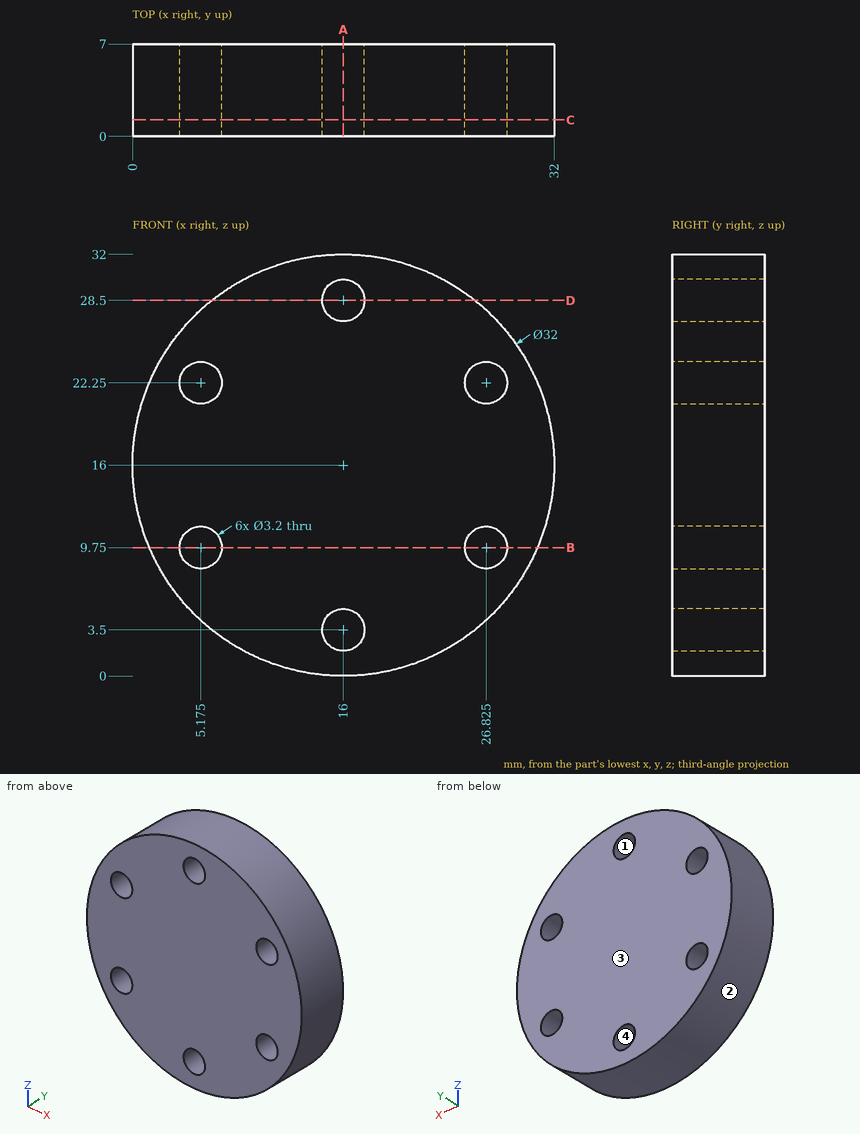
Source: three-view drawing plus pictorial views. Frame: mm from the lowest corner of the part. Give positions to 0.01 mm unless a question says otherwise; leave off trailing zeros. Write each loop counter-clockwise with the first axis right and the second up, starting at its lowest first coordinate (ties: lowest second). Pieces come first, ordered by that corner, then holes. Notation, with made-up numbers: (8, 38) -> (33, 38) arc R25 ccw to (33, 56) -> close; hole circle Ø5 at (-30, -8.75). An arc over 180 degrees is marked (long way). Answer in a Markdown table with one row per item.
(1) Ray query, line 1 along Z through (x, y) = (4.5, 5.25) (1 decimal); line 2 along Z through (x, y) = (26, 5); line 3 along X through (y, z) = (5.25, 4) (1 decimal). Return the intervals inside material, ascending. Write a range as [from, to].
Answers below:
| item | result |
|---|---|
| line 1 | [4.9, 8.3], [11.2, 20.8], [23.7, 27.1] |
| line 2 | [3.51, 8.38], [11.12, 20.88], [23.62, 28.49] |
| line 3 | [5.4, 14.5], [17.5, 26.6] |
(2) Section query D-D on z = 28.5. Return loops of the section in (x, y).
Answers below:
| item | result |
|---|---|
| outline | (6.01, 0) -> (14.4, 0) -> (14.4, 7) -> (6.01, 7) -> close; (17.6, 0) -> (25.99, 0) -> (25.99, 7) -> (17.6, 7) -> close |
(3) Draft query along Z for the marked faces 1, 2, 3 and 4. Return one class per face: +Z half, -Z half, draft (parallel to the pull), parting line (faces both ways), or undercut.
Answers below:
| item | result |
|---|---|
| face 1 | undercut |
| face 2 | parting line |
| face 3 | draft |
| face 4 | undercut |
(4) Section query A-A on x = 16. Return loops of the section in (y, z), then the cut area to 3 significant figures.
Answers below:
| item | result |
|---|---|
| outline | (0, 0) -> (7, 0) -> (7, 1.9) -> (0, 1.9) -> close; (0, 5.1) -> (7, 5.1) -> (7, 26.9) -> (0, 26.9) -> close; (0, 30.1) -> (7, 30.1) -> (7, 32) -> (0, 32) -> close |
| area | 179 mm^2 |
(5) Section query C-C on y = 1.25. State how many separate pieces and enclosed holes the cut face has, then the cut area to 3 significant figures.
Answers below:
| item | result |
|---|---|
| separate pieces | 1 |
| enclosed holes | 6 |
| area | 756 mm^2 |
(6) Section query B-B on z = 9.75. Return loops of the section in (x, y) (1 decimal).
Answers below:
| item | result |
|---|---|
| outline | (1.3, 0) -> (3.6, 0) -> (3.6, 7) -> (1.3, 7) -> close; (6.8, 0) -> (25.2, 0) -> (25.2, 7) -> (6.8, 7) -> close; (28.4, 0) -> (30.7, 0) -> (30.7, 7) -> (28.4, 7) -> close |
(7) Pin query (flat end, axial travel): pin 1 (4 mm diameter, centred on x = 16, z = 28.5, fed in from -Y); pin 2 (2 mm diameter, centred on y = 6, z = 23, fed in from +X); pin 3 (2 mm diameter, centred on y = 6, z = 10.5, fed in from -X). Return the tip coordinate at first contact, or that it passes through.
Answers below:
| item | result |
|---|---|
| pin 1 | y = 0 |
| pin 2 | x = 30.83 |
| pin 3 | x = 0.65 |
